The drawing under review shows one solid part. Ordinate dimensions are in mm from its lowest x, y, z. A direction names the side the tool comes from. Round coordinates to 2 decimals unless told otherwise and drop trailing zeros. Order: outer loops, then holes, each group sorted by start corner. A loop starts at its lowest first (then second) coordinate and runs counter-clockwise, first axis right, second up. Notation, with made-up numbers: M -10,-13 L 23,-13 A5 cw 23,-8 Z; hole C -4,73.5 d9. An arc over 180 degrees is marked long. Use a Markdown table: item, result.
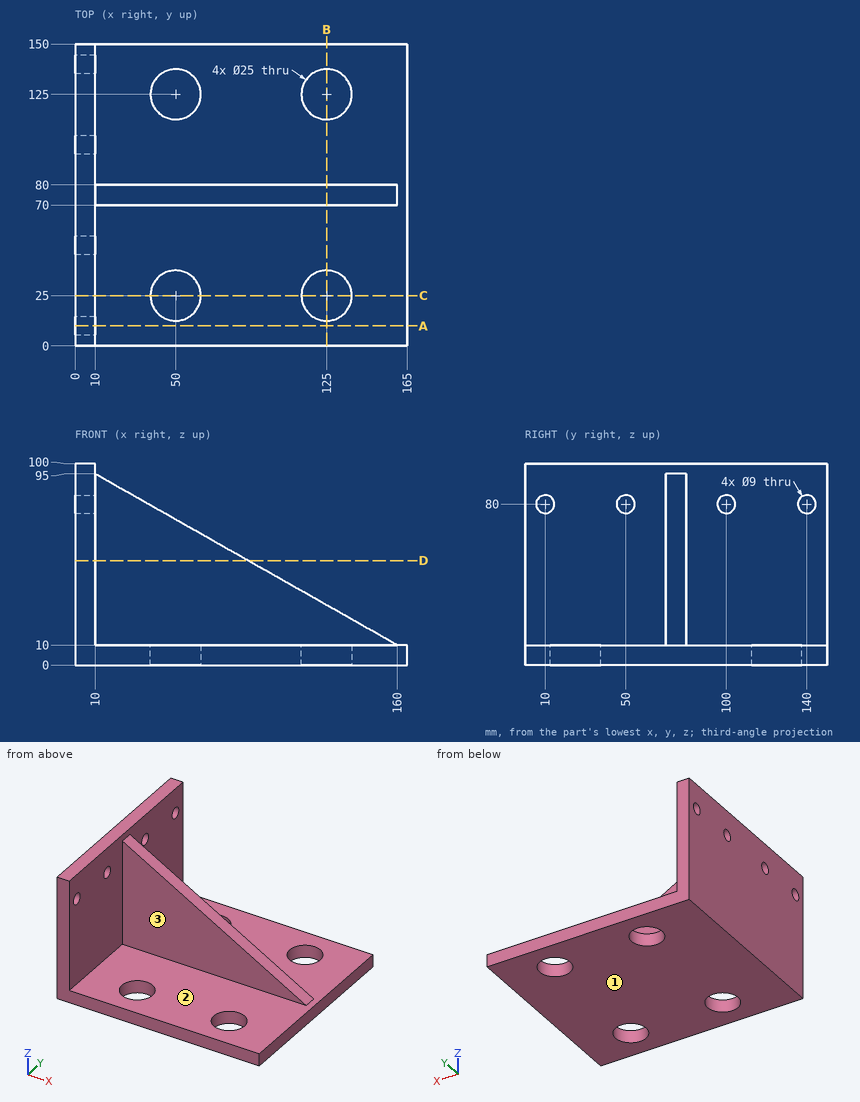
Q1. Wall thickness on line 1 along Y through (x, z) = (50, 8); line 2 along Z through (x, y) = (7, 50); line 3 along X through (y, z) = (84, 40): over which ranges is each line inside the solid? List them lowest first. Write a range as [from, to].
Determined:
| item | result |
|---|---|
| line 1 | y = [0, 12.5], [37.5, 112.5], [137.5, 150] |
| line 2 | z = [0, 75.5], [84.5, 100] |
| line 3 | x = [0, 10] |
Q2. Add section D-D (z = 52). Write out the cut boundary in (x, y).
Determined:
| item | result |
|---|---|
| outline | M 0,0 L 10,0 L 10,70 L 85.88,70 L 85.88,80 L 10,80 L 10,150 L 0,150 Z |
Q3. Clearance check with flat-ended pins moving along their axes: pin 1 (1.5 mm diameter, centred on x = 78.5, z = 22, fed in from -Y); pin 2 (15 mm diameter, centred on x = 125, y = 25, fed in from -Z); pin 3 (5 mm diameter, centred on x = 84.5, y = 74, fed in from +Z); pin 4 (10.5 mm diameter, centred on y = 100, z = 80, fed in from +X). State where each tip first meets the part, or that it passes through.
Determined:
| item | result |
|---|---|
| pin 1 | stops at y = 70 |
| pin 2 | passes through |
| pin 3 | stops at z = 54.2 |
| pin 4 | stops at x = 10 |
Q4. Machinability: for the marked faces 1, 2 and 3, which of the approach directions +Z, -Z, +X, -X, +Y, -Y give a long, thin tool a straight path to every point of the face, cutting with its end or side? Answer none if there is none.
Determined:
| item | result |
|---|---|
| face 1 | -Z, +X, -X, +Y, -Y |
| face 2 | +Z, +X |
| face 3 | +Z, +X, -Y |
Q5. Add section A-A (y = 10). Write out the cut boundary in (x, z), then the cut area to 3 significant figures.
Determined:
| item | result |
|---|---|
| outline | M 0,0 L 165,0 L 165,10 L 10,10 L 10,75.5 L 0,75.5 Z; M 0,84.5 L 10,84.5 L 10,100 L 0,100 Z |
| area | 2,460 mm^2 |
Q6. Add section B-B (x = 125). Write out the cut boundary in (y, z), then the cut area to 3 significant figures.
Determined:
| item | result |
|---|---|
| outline | M 0,0 L 12.5,0 L 12.5,10 L 0,10 Z; M 37.5,0 L 112.5,0 L 112.5,10 L 80,10 L 80,29.83 L 70,29.83 L 70,10 L 37.5,10 Z; M 137.5,0 L 150,0 L 150,10 L 137.5,10 Z |
| area | 1,200 mm^2 |
Q7. Add section C-C (y = 25). Write out the cut boundary in (x, z).
Determined:
| item | result |
|---|---|
| outline | M 0,0 L 37.5,0 L 37.5,10 L 10,10 L 10,100 L 0,100 Z; M 62.5,0 L 112.5,0 L 112.5,10 L 62.5,10 Z; M 137.5,0 L 165,0 L 165,10 L 137.5,10 Z |
